The drawing under review shows one solid part. Ordinate dimensions are in mm from its lowest x, y, z. A direction names the side the tool comes from. Coordinates: 2 decimals unless noted, no trailing zeros. Order: outer loops, then holes, each group sorted by start corner. A loop starts at its lowest first (then second) coordinate and runs counter-clockwise, first axis right, second up. Notation, with made-up numbers: (46.5, 42.25) -> (89.5, 42.25) arc R19 cw to (89.5, 52.25) -> close; hole circle Ø3 at (41, 9.5). An arc over 180 degrees is marked (long way). Write item = value, one per line.
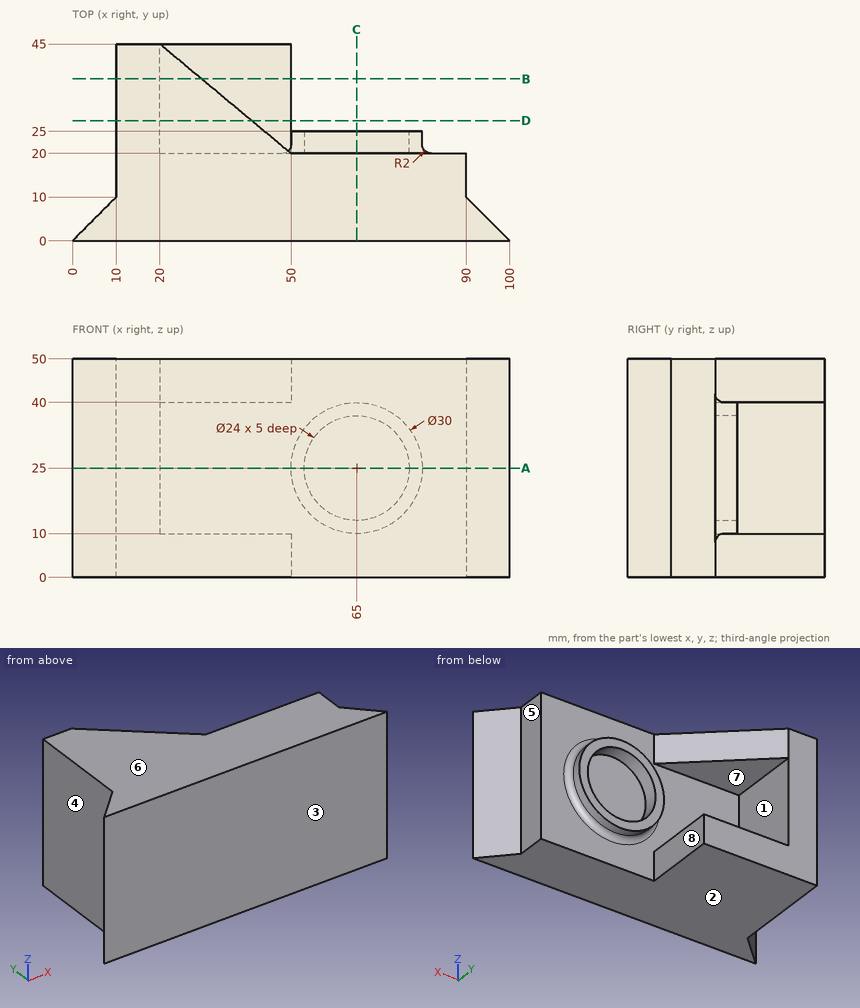
(1) For L1, parallel to X at y = 22.35, z = 25; L2, parallel to Z at x = 65, y = 22.4; L3, parallel to X at y = 21.55, z = 25, list the stretches that pass through material, from the lowest coordinate up.
Report:
L1 = 10 to 20, 50 to 53, 77 to 80
L2 = 10 to 13, 37 to 40
L3 = 10 to 20, 49.95 to 53, 77 to 80.05
(2) Insertion check: pin 1 (24 mm diameter, centred on x = 72, z = 19.5, fed in from +Y); pin 2 (5 mm diameter, centred on y = 16, z = 29, fed in from +X); pin 3 (2 mm diameter, centred on y = 27, z = 38, fed in from +X). Each pin has a flat end and moves straight along its axis. Give the tip position at first contact, or say it passes through.
Report:
pin_1 = 25
pin_2 = 90
pin_3 = 20
(3) We need section B-B (y = 37). Write out the cut boundary in (x, z), and give its area (3 significant figures).
Report:
outline = (10, 0) -> (50, 0) -> (50, 10) -> (20, 10) -> (20, 40) -> (29.6, 40) -> (29.6, 50) -> (10, 50) -> close
area = 896 mm²
(4) The part is to be moulded in two halves that separate along Z. For the marked faces 6, 7 and 8, say which applies: released by +Z, released by -Z, zero draft, split by the parting line, or undercut.
Report:
face_6 = released by +Z
face_7 = undercut
face_8 = zero draft
(5) We need section D-D (y = 27.5). Write out the cut boundary in (x, z), and give its area (3 significant figures).
Report:
outline = (10, 0) -> (50, 0) -> (50, 10) -> (20, 10) -> (20, 40) -> (41, 40) -> (41, 50) -> (10, 50) -> close
area = 1,010 mm²
(6) We need section A-A (z = 25). Write out the cut boundary in (x, y).
Report:
outline = (0, 0) -> (100, 0) -> (90, 10) -> (90, 20) -> (82, 20) arc R2 cw to (80, 22) -> (80, 25) -> (77, 25) -> (77, 20) -> (53, 20) -> (53, 25) -> (50, 25) -> (50, 22) arc R2 cw to (48, 20) -> (20, 20) -> (20, 45) -> (10, 45) -> (10, 10) -> close
(7) We need section C-C (x = 65). Write out the cut boundary in (y, z), and give its area (3 significant figures).
Report:
outline = (0, 0) -> (20, 0) -> (20, 8) arc R2 cw to (22, 10) -> (25, 10) -> (25, 13) -> (20, 13) -> (20, 37) -> (25, 37) -> (25, 40) -> (22, 40) arc R2 cw to (20, 42) -> (20, 50) -> (0, 50) -> close
area = 1,030 mm²
(8) For the marked faces 1, 2, 3, 4 and 5, list the 3-axis set-ups (+Z, -Z, +X, -X, +Y, -Y) from which the entire face can be reached by the end or side of a thin tool; tool diameter is ignored.
Report:
face_1 = +Y
face_2 = -Z, +X, -X, +Y, -Y
face_3 = +Z, -Z, +X, -X, -Y
face_4 = +Z, -Z, -X, +Y
face_5 = +Z, -Z, +X, +Y
